```python
from build123d import *

# Parameters (mm, degrees)
BOSS_EXTRUDE1_DEPTH = 3
SKETCH3_W           = 3
SKETCH3_H           = 20
BOSS_EXTRUDE2_DEPTH = 3


with BuildPart() as part:
    # Sketch1 → Boss-Extrude1 (new body)
    with BuildSketch(Plane.XY):
        Polygon((-204, 9), (-204, 6), (-225, 6), (-225, 72), (-204, 72), (-204, 69), (-180, 69), (-180, 72), (-156, 72), (-156, 69), (-132, 69), (-132, 72), (-108, 72), (-108, 69), (-84, 69), (-84, 72), (-60, 72), (-60, 69), (-36, 69), (-36, 72), (-12, 72), (-12, 69), (12, 69), (12, 72), (36, 72), (36, 69), (60, 69), (60, 72), (84, 72), (84, 69), (108, 69), (108, 72), (132, 72), (132, 69), (156, 69), (156, 72), (180, 72), (180, 69), (204, 69), (204, 72), (225, 72), (225, 6), (204, 6), (204, 9), (180, 9), (180, 6), (156, 6), (156, 9), (132, 9), (132, 6), (108, 6), (108, 9), (84, 9), (84, 6), (60, 6), (60, 9), (36, 9), (36, 6), (12, 6), (12, 9), (-12, 9), (-12, 6), (-36, 6), (-36, 9), (-60, 9), (-60, 6), (-84, 6), (-84, 9), (-108, 9), (-108, 6), (-132, 6), (-132, 9), (-156, 9), (-156, 6), (-180, 6), (-180, 9), align=None)
    extrude(amount=BOSS_EXTRUDE1_DEPTH)

    # Sketch3 → Boss-Extrude2 (add)
    with BuildSketch(Plane.XY.offset(3)):
        with Locations((-226.5, 59)):
            Rectangle(SKETCH3_W, SKETCH3_H)
        with Locations((-226.5, 19)):
            Rectangle(SKETCH3_W, SKETCH3_H)
        with Locations((226.5, 59)):
            Rectangle(SKETCH3_W, SKETCH3_H)
        with Locations((226.5, 19)):
            Rectangle(SKETCH3_W, SKETCH3_H)
    extrude(amount=-BOSS_EXTRUDE2_DEPTH)


solid = part.part
```
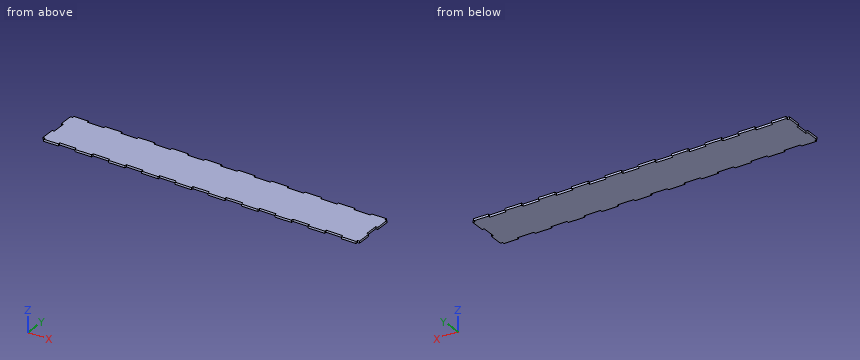
Here's how the part is built. I have some questions about the finished solid (model axes, mm). Coordinates: 2 decimals unless noted, no trailing zeros. Order: outer loops, then holes, each group sorted by start corner. A loop starts at its lowest first (then second) coordinate and runs counter-clockwise, first axis right, second up. Notation, with made-up numbers: (-7, 78.25) - (25, 78.25) arc R15 ccw to (25, 85.25) - close; hole circle Ø7 at (32.25, 86.25). An arc over 180 degrees is marked (long way). One line per question, with ' | ' between items.
(1) Suppose I cut it at A-A on x = -51. List the corners of the cut face in (y, z) for me, and give its area (3 significant figures).
Report:
outline: (9, 0) - (69, 0) - (69, 3) - (9, 3) - close | area: 180 mm2
(2) Will these pins go through, and if not, where does the flat tip stop? pin 1 (1.5 mm diameter, centred on x = -147.5, z = 1, fed in from -Y); pin 2 (1.5 mm diameter, centred on y = 7, z = 1, fed in from -X); pin 3 (1.5 mm diameter, centred on y = 7, z = 1.5, fed in from +X).
Report:
pin 1: stops at y = 9 | pin 2: stops at x = -225 | pin 3: stops at x = 225
(3) If I drill on L1, parallel to Y at x = -59.5, z = 2.4; L2, parallel to X at y = 40, z = 2.1, over which ranges is the centre line in solid material (lowest first)?
Report:
L1: y = 9 to 69 | L2: x = -225 to 225
